Autodesk Inventor part; units mm, degrees
ref_plane "YZ Plane" through (0, 0, 0) normal (1, 0, 0) x (0, 1, 0)
ref_plane "XZ Plane" through (0, 0, 0) normal (0, 1, 0) x (-1, 0, 0)
ref_plane "XY Plane" through (0, 0, 0) normal (0, 0, 1) x (1, 0, 0)
sketch "Эскиз1" plane through (0, 0, 0) normal (0, 0, 1) x (1, 0, 0)
  line L0 (0, 0) -> (45, 0)
  line L1 (45, 0) -> (45, -45)
  line L2 (45, -45) -> (35, -45)
  line L3 (20, -65) -> (20, 0)
  line L4 (35, -45) -> (27.6938, -65.0737)
  line L5 (20, -57.4838) -> (30.4563, -57.4838)
  line L6 (0, 0) -> (0, -13.3093)
  dimension "d0" = 45
  dimension "d1" = 45
  dimension "d2" = 10
  dimension "d5" = 20
  dimension "d6" = 110
revolve "Вращение1" add sketch "Эскиз1" angle 360 about axis through (0, 0, 0) along (0, -1, 0)
thread "Резьба1"
chamfer "Фаска1" distance 2 angle 45 2 edges at (-20, 0, 0) (-20, -57.4838, 0)
sketch "Эскиз2" plane through (0, 0, 0) normal (0, 0, 1) x (1, 0, 0)
  line L0 (45, 0) -> (45, -45)
  line L1 (45, 0) -> (45, -15)
  line L2 (45, -15) -> (34.4215, -15)
  line L3 (45, -15) -> (45, -10)
  line L4 (45, -10) -> (35, -10)
  line L5 (35, -10) -> (31.8757, -15)
  line L6 (34.4215, -15) -> (31.8757, -15)
  point P0 (0, 0)
  dimension "d13" = 15
  dimension "d14" = 5
  dimension "d15" = 10
  dimension "d17" = 58
revolve "Вращение2" cut sketch "Эскиз2" angle 360 about axis through (45, -15, 0) along (-1, 0, 0)
properties part number "Гайка шток-поршень" material "Сталь, углеродистая"
Part model, mm, in its own coordinate system. A direction names the side the tool comes from. Coordinates: 2 decimals unless noted, no trailing zeros. Loops run counter-clockwise (first coordinate to the right, second up) from the corner with the lowest first, then second, coordinate; pieces in that order, holes last. Notation, with made-up numbers: (83.5, 1.25) - (142.5, 1.25) arc R26 cw to (142.5, 33.25) - close; hole circle Ø10 at (45.25, 81). An arc over 180 degrees is marked (long way). Write item = value, one per line. Start each with the question number.
Item 1: Cut at A-A, the plane y = -22.5. Give the cut face in (x, z), and give its area (3 significant figures).
Item 2: Cut at C-C, the plane y = -50. Give the cut face in (x, z), and give its area (3 significant figures).
Item 3: Mould opens along X. For faces 4 (the cylindrical face through (20.765, -22.815, -39.923)), 5 (the flat face through (9, 0, 21)), 6 (the conical face through (-4.36, -1.87, 19.65)) say: released by +X, released by -X, zero draft, split by the parting line, or undercut.
Item 4: Wall check: L1, parallel to Z at x = 0, y = -19; L2, parallel to Y at x = 38, z = 0; L3, parallel to X at y = -50.5, z = -15.5. Give the ranges that are in metal, low to high. Write a range as from..to.
Item 5: Flat gauge pins, fed straight in: pin 1 Ø3 at (x, z) = (-29, 9.5) entering from -Y; pin 2 Ø10 at (x, y) = (-21, -18) entering from +Z; pin 3 Ø8 at (y, z) = (-40.5, -26.5) entering from +X; pin 4 Ø5 at (y, z) = (-37, -23) entering from +X. Where does each tip first touch, or does it go through?
Item 6: 3-axis set-ups, long thin cutter, end or side, ignore diameter. For faces 1 (the flat face through (23.1, -45, -26.5)), 2 (the cylindrical face through (-4.336, -28.368, 19.524)), 3 (the cylindrical face through (40, -20, 0)): which of +Z, -Z, +X, -X, +Y, -Y reach the whole face in a straight line?
Item 7: Cut at B-B, the plane x = 0. Give the cut face in (y, z).
The answers:
q1.outline = circle Ø90 at (0, 0); hole circle Ø40 at (0, 0)
q1.area = 5,110 mm2
q2.outline = circle Ø66.36 at (0, 0); hole circle Ø40 at (0, 0)
q2.area = 2,200 mm2
q3.face_4 = split by the parting line
q3.face_5 = zero draft
q3.face_6 = undercut
q4.L1 = -45..-20, 20..45
q4.L2 = -45..-20, -10..0
q4.L3 = -29.13..-12.64, 12.64..29.13
q5.pin_1 = -57.48
q5.pin_2 = 42.06
q5.pin_3 = 38.97
q5.pin_4 = 40.06
q6.face_1 = -Y
q6.face_2 = +Y, -Y
q6.face_3 = +X
q7.outline = (-57.48, -30.46) - (-45, -35) - (-45, -45) - (0, -45) - (0, -22) - (-2, -20) - (-55.48, -20) - (-57.48, -22) - close; (-57.48, 22) - (-55.48, 20) - (-2, 20) - (0, 22) - (0, 45) - (-45, 45) - (-45, 35) - (-57.48, 30.46) - close
